The listing builds one solid part. Answer for the finished solid, in the listing's coordinates (mm). Face numbers are marked on the shaded views. A direction names the side the tool comes from. Give positions to 0.01 mm unless a question says otherwise; leave off trailing zeros. Write each loop counter-clockwise with the first axis right and the second up, starting at its lowest first coordinate (ties: lowest second). Pieces come first, ordered by that corner, then holes. Notation, with made-up numbers: M 61.25,60.25 L 88.25,60.25 A19 cw 88.25,80.25 Z; hole C -9.75,12.5 d11. An arc over 180 degrees is marked long. Return JSON: item names as keys, results as strings.
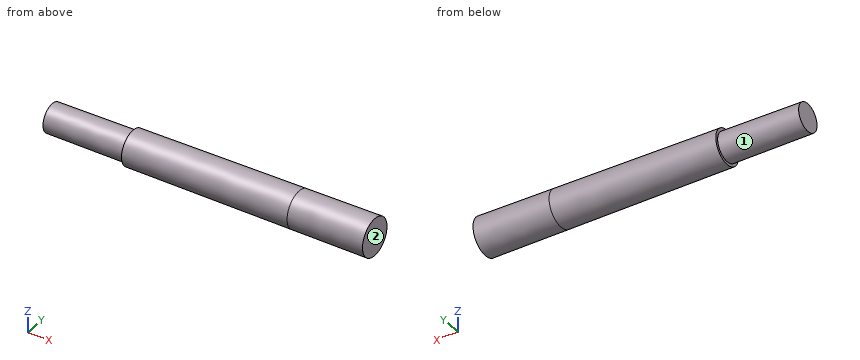
from build123d import *


with BuildPart() as f2:
    # F1 (on Top) → F2 (revolve)
    with BuildSketch(Plane.XY):
        Polygon((31.9, 0), (48.9, 0), (48.9, 3.073067), (31.903461, 2.97501), align=None)
        Polygon((48.9, 0), (83.9, 0), (83.9, 3.875), (48.9, 3.673077), (48.903461, 3.073087), (48.9, 3.073067), align=None)
        Polygon((83.9, 3.875), (83.9, 0), (99.855002, 0), (99.855002, 3.967048), align=None)
    revolve(axis=Axis((24.45, 0, 0), (1, 0, 0)))


solid = f2.part
Item 1: Find the intervals of material crossed by line 1 (X direction, y = 1.5, z = -1) (3 decimals); line 2 (Z direction, x = 89, y = -0.5); line 3 (X direction, y = -1, z = 3.5) (3 decimals), in increasing order.
Geometry results:
{"line 1": "x = 31.902 to 99.855", "line 2": "z = -3.87 to 3.87", "line 3": "x = 48.9 to 99.855"}
Item 2: Given pin 1 Ø2 at (x, y) = (83.5, 1.5) entering from +Z, flat-ended and moving along its own axis, determine where the tip first touches the part or whether it passes through.
Geometry results:
{"pin 1": "stops at z = 3.84"}
Item 3: Which of the six approach directions +Z, -Z, +X, -X, +Y, -Y give full straight-line access (tool end or side, diameter ignored) to the marked faces 1 and 2?
Geometry results:
{"face 1": "-X", "face 2": "+Z, -Z, +X, +Y, -Y"}
Item 4: A cutting plane is placed at B-B, the plane x = 50. Write down the section's boundary in (y, z).
Geometry results:
{"outline": "C 0,0 d7.36"}
Item 5: A cutting plane is placed at A-A, the plane x = 39.5. Write down the section's boundary in (y, z), plus the area to 3 significant figures.
Geometry results:
{"outline": "C 0,0 d6.04", "area": "28.6 mm2"}
